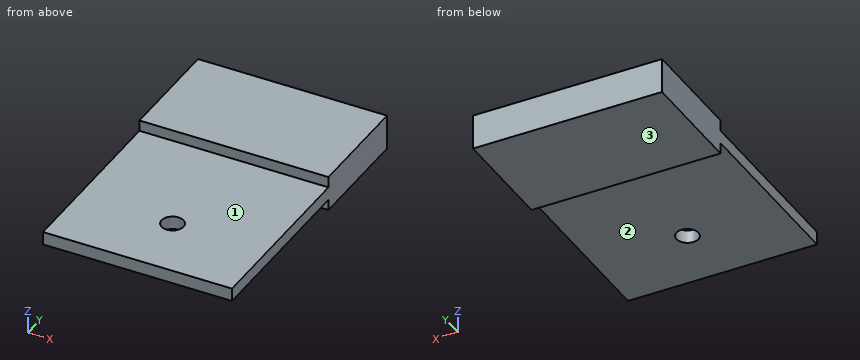
from build123d import *

# Parameters (mm, degrees)
SKETCH1_W           = 86.202021521
SKETCH1_H           = 82.381948497
SKETCH1_R           = 5
BOSS_EXTRUDE1_DEPTH = 6
BOSS_EXTRUDE2_DEPTH = 50


with BuildPart() as part:
    # Sketch1 → Boss-Extrude1 (new body)
    with BuildSketch(Plane.XY):
        with Locations((-54.060241917, 22.740820087)):
            Rectangle(SKETCH1_W, SKETCH1_H)
        with Locations((-54.060241916, 11.48296308)):
            Circle(SKETCH1_R, mode=Mode.SUBTRACT)
    extrude(amount=BOSS_EXTRUDE1_DEPTH)

    # Sketch2 → Boss-Extrude2 (add)
    with BuildSketch(Plane(origin=(0, 63.931794335, 0), x_dir=(1, 0, 0), z_dir=(0, 1, 0))):
        Polygon((-97.161252677, -6), (-97.161252677, -11), (-10.959231156, -11), (-10.959231156, 5), (-97.161252677, 5), align=None)
    extrude(amount=BOSS_EXTRUDE2_DEPTH)


solid = part.part
Read the model definition and answer for the solid it produces. Units are mm, in the model's axes. Face numbers are marked on the shaded views. A direction names the side the tool comes from. Coordinates: 2 decimals unless noted, no trailing zeros. Order: outer loops, then holes, each group sorted by start corner. A loop starts at its lowest first (then second) coordinate and runs counter-clockwise, first axis right, second up. Notation, with made-up numbers: (71.25, 21) -> (130.25, 21) arc R17 cw to (130.25, 38) -> close; hole circle Ø1 at (72.25, -16). An arc over 180 degrees is marked (long way). Answer as a JSON object with one key per item and string values.
1) A cutting plane is placed at C-C, the plane y = 2.5. Determine the outline of the cut face in (x, z).
Model answer:
{"outline": "(-97.16, 0) -> (-10.96, 0) -> (-10.96, 6) -> (-97.16, 6) -> close"}
2) Consider line 1 along X through (y, z) = (11, 4.5); line 2 along Y through (x, z) = (-73.5, -1.25); line 3 along Z through (x, y) = (-79, 17.5). Determine where each line is inside the solid, lowest interval first. Write a range as from..to.
Model answer:
{"line 1": "x = -97.16..-59.04, -49.08..-10.96", "line 2": "y = 63.93..113.93", "line 3": "z = 0..6"}
3) A cutting plane is placed at B-B, the plane z = 8.5. Determine the outline of the cut face in (x, y), plus the area to 3 significant figures.
Model answer:
{"outline": "(-97.16, 63.93) -> (-10.96, 63.93) -> (-10.96, 113.93) -> (-97.16, 113.93) -> close", "area": "4,310 mm²"}
4) A tool of negligible diameter and unlimited length cuts with its end or side. For the marked faces 1, 2 and 3, from which of +Z, -Z, +X, -X, +Y, -Y can it reach the whole face along a straight path? Write none if from no direction.
Model answer:
{"face 1": "+Z, +X, -X, -Y", "face 2": "-Z, +X, -X, -Y", "face 3": "-Z, +X, -X, +Y, -Y"}
5) Each of these flat-tipped pins is pushed along its axis until it touches: pin 1 (1.5 mm diameter, centred on x = -45, z = -1.5, fed in from -Y); pin 2 (11.5 mm diameter, centred on x = -54.06, y = 11.48, fed in from -Z). Where does it stop, or does it pass through?
Model answer:
{"pin 1": "stops at y = 63.93", "pin 2": "stops at z = 0"}
6) A cutting plane is placed at A-A, the plane x = -70. Determine the outline of the cut face in (y, z).
Model answer:
{"outline": "(-18.45, 0) -> (63.93, 0) -> (63.93, -5) -> (113.93, -5) -> (113.93, 11) -> (63.93, 11) -> (63.93, 6) -> (-18.45, 6) -> close"}
